from build123d import *

# Parameters (mm, degrees)
SKETCH1_W           = 12
SKETCH1_H           = 4
CHAMFER1_SIZE       = 0.9375
SKETCH11_R          = 8.9
BOSS_EXTRUDE3_DEPTH = 1.1
CUT_EXTRUDE2_DEPTH  = 3.08


with BuildPart() as part:
    # Sketch1 → Revolve1 (revolve)
    with BuildSketch(Plane(origin=(0, 0, 0), x_dir=(0, 0, -1), z_dir=(1, 0, 0))):
        with Locations((10.4, 2)):
            Rectangle(SKETCH1_W, SKETCH1_H)
    revolve(axis=Axis((0, 0, -16.4), (0, 0, 1)))

    # Chamfer1
    chamfer1_edges = [part.edges().sort_by_distance(p)[0] for p in [
        (0, -4, -16.4),
    ]]
    chamfer(chamfer1_edges, length=CHAMFER1_SIZE)

    # Sketch7 → Revolve2 (revolve)
    with BuildSketch(Plane(origin=(0, 0, 0), x_dir=(0, 0, -1), z_dir=(1, 0, 0)), mode=Mode.PRIVATE) as revolve2_sk:
        with BuildLine():
            Line((3.3, 6.5), (4.4, 6.5))
            Line((4.4, 6.5), (4.4, 0))
            Line((4.4, 0), (0, 0))
            Line((0, 0), (0, 4))
            ThreePointArc((0, 4), (1.458196289, 5.503180898), (3.3, 6.5))
        make_face()
    revolve(revolve2_sk.sketch.rotate(Axis((0, 0, 0), (0, 0, -1)), 180), axis=Axis((0, 0, 0), (0, 0, -1)))

    # Sketch11 → Boss-Extrude3 (add)
    with BuildSketch(Plane(origin=(0, 0, -4.4), x_dir=(-1, 0, 0), z_dir=(0, 0, -1))):
        Circle(SKETCH11_R)
    extrude(amount=-BOSS_EXTRUDE3_DEPTH)

    # Sketch5 → Cut-Extrude2 (cut)
    with BuildSketch(Plane.XY):
        Polygon((2.5, -1.443375673), (2.5, 1.443375673), (0, 2.886751346), (-2.5, 1.443375673), (-2.5, -1.443375673), (0, -2.886751346), align=None)
    extrude(amount=-CUT_EXTRUDE2_DEPTH, mode=Mode.SUBTRACT)

    # Cut-Extrude3 cone 1 section (through the dimple's axis) → Cut-Extrude3 (revolve, cut)
    with BuildSketch(Plane(origin=(0, 0, 0), x_dir=(0, -1, 0), z_dir=(1, 0, 0))):
        Polygon((0, 0), (2.886751346, 0), (0, 2.886751346), align=None)
    revolve(axis=Axis((0, 0, 0), (0, 0, -1)), mode=Mode.SUBTRACT)


solid = part.part
Geometry: final body of the model. Coordinates: model frame, mm. A direction names the side the tool comes from. Round coordinates to 2 decimals unless told otherwise and drop trailing zeros. Order: outer loops, then holes, each group sorted by start corner. A loop starts at its lowest first (then second) coordinate and runs counter-clockwise, first axis right, second up. Notation, with made-up numbers: (42.5, -37.75) - (53.5, -37.75) arc R18 ccw to (53.5, -21.75) - close; hole circle Ø8 at (57.5, 83). An arc over 180 degrees is marked (long way). Write each question's results on one line, items separated by ' | '.
Item 1: Mould query, pull axis X, two halves, no side actions, for faces 4 (the cylindrical face through (3.905, -0.867, -10.009)), 5 (the flat face through (0, 0, -16.4)), 6 (the conical face through (-1.328, -2.34, -0.196)). Classes: pulls with the +X half, pulls with the -X half, needs draft (parallel to the pull), parting line crosses it, or undercut.
Completed:
face 4: parting line crosses it | face 5: needs draft | face 6: undercut
Item 2: Material intervals for line 1 along Z through (x, y) = (-1.5, -0.5); line 2 along X through (y, z) = (0, -1.5); line 3 along Z through (x, y) = (-7.5, 2), sorted ascending. Write a range as [from, to].
Completed:
line 1: [-16.4, -3.08] | line 2: [-5.53, -2.5], [2.5, 5.53] | line 3: [-4.4, -3.3]
Item 3: Section A-A, the plane y = 0. Return the cut outline in (x, z), and give its area (3 significant figures).
Completed:
outline: (-8.9, -4.4) - (-4, -4.4) - (-4, -15.46) - (-3.06, -16.4) - (3.06, -16.4) - (4, -15.46) - (4, -4.4) - (8.9, -4.4) - (8.9, -3.3) - (6.5, -3.3) arc R6.9 ccw to (4, 0) - (2.89, 0) - (2.5, -0.39) - (2.5, -3.08) - (-2.5, -3.08) - (-2.5, -0.39) - (-2.89, 0) - (-4, 0) arc R6.9 ccw to (-6.5, -3.3) - (-8.9, -3.3) - close | area: 136 mm^2
Item 4: Section D-D, the plane z = -10. Return the cut outline in (x, y), and give its area (3 significant figures).
Completed:
outline: circle Ø8 at (0, 0) | area: 50.3 mm^2
Item 5: Section B-B, the plane z = -0.75. Return the cut outline in (x, y), and give its area (3 significant figures).
Completed:
outline: circle Ø9.77 at (0, 0); hole (-2.5, -1.44) - (0, -2.89) - (2.5, -1.44) - (2.5, 1.44) - (0, 2.89) - (-2.5, 1.44) - close | area: 53.4 mm^2
Item 6: Reachability of faces 1 (the cylindrical face through (1.93, -8.69, -3.86)), 2 (the flat face through (-4, -2, -4.4)), 3 (the conical face through (1.36, -2.32, -0.2)) from +Z, -Z, +X, -X, +Y, -Y: full face, straight path, thin tool, end or side. Return the list, or none.
Completed:
face 1: +Z, -Z | face 2: -Z | face 3: +Z
Item 7: First-contact query: pin 1 Ø1.5 at (x, y) = (5, 1.5) entering from -Z; pin 2 Ø2.5 at (y, z) = (-0.5, -2) entering from -X; pin 3 Ø0.9 at (y, z) = (0, -2) entering from +X. Flat tips, straight axial feed; report the tip coordinate or a pass-through.
Completed:
pin 1: z = -4.4 | pin 2: x = -6.47 | pin 3: x = 6.13
Item 8: Section C-C, the plane x = 5.5. Return the cut outline in (y, z), and give its area (3 significant figures).
Completed:
outline: (-7, -4.4) - (7, -4.4) - (7, -3.3) - (3.46, -3.3) arc R4.17 ccw to (-3.46, -3.3) - (-7, -3.3) - close | area: 24.4 mm^2
